Geometry check sheet. Reference: the model listing, model coordinates, mm. Give positions to 0.01 mm unless a question says otherwise; leave off trailing zeros. Write each loop counter-clockwise with the first axis right and the second up, starting at its lowest first coordinate (ties: lowest second). Pieces come first, ordered by that corner, then holes. Notation, with made-up numbers: M 41.5,36 L 54.5,36 A13 cw 54.5,54 Z; hole C 84,-3 d10. An arc over 180 degrees is marked long. One line per item, written item: value. Start each with the question number.
1. Cross-section at C-C on y = 264.5. Record the cut outline in (x, z), then the cut area to 3 significant figures.
2. Gauge pin test, flat ends, axial feed: pin 1 (10 mm diameter, centred on x = 123, z = -49.5, fed in from -Y); pin 2 (1 mm diameter, centred on x = -115, z = -49, fed in from +Y); pin 3 (3 mm diameter, centred on x = -211, z = 49.5, fed in from +Y). Record the tip position at first contact, or that the pin passes through.
3. Cross-section at A-A on z = -48.5. Record the cut outline in (x, y), then the cut area to 3 significant figures.
4. Cross-section at D-D on z = 40. Record the cut outline in (x, y), then the cut area to 3 significant figures.
5. Cross-section at B-B on x = 142. Record the cut outline in (y, z), then the cut area to 3 significant figures.
6. Scan lines: line 1 (Y direction, x = 126.5, z = 22); line 2 (Y direction, x = -320, z = -19). Record each from-to range of solid material in increasing order.
Autodesk Inventor part; units mm, degrees
ref_plane "YZ Plane" through (0, 0, 0) normal (1, 0, 0) x (0, 1, 0)
ref_plane "XZ Plane" through (0, 0, 0) normal (0, 1, 0) x (-1, 0, 0)
ref_plane "XY Plane" through (0, 0, 0) normal (0, 0, 1) x (1, 0, 0)
sketch "Sketch1" plane through (0, 0, 0) normal (0, 1, 0) x (-1, 0, 0)
  line L0 (431.8, -82.55) -> (-431.8, -82.55)
  line L1 (-431.8, -82.55) -> (-431.8, 82.55)
  line L2 (-431.8, 82.55) -> (431.8, 82.55)
  line L3 (431.8, 82.55) -> (431.8, -82.55)
  line L4 (431.8, -82.55) -> (-431.8, 82.55) construction
  line L5 (-431.8, -82.55) -> (431.8, 82.55) construction
  point P0 (0, 0)
  dimension "d0" = 863.6
  dimension "d1" = 165.1
extrude "Extrusion1" add sketch "Sketch1" along normal blind 304.8
sketch "Sketch2" plane through (431.8, 0, 82.55) normal (1, 0, 0) x (0, 0, -1)
  line L0 (0, 304.8) -> (165.1, 304.8)
  line L1 (165.1, 0) -> (165.1, 304.8)
  line L2 (12.7, 304.8) -> (165.1, 254)
  line L3 (165.1, 254) -> (165.1, 304.8)
  line L4 (165.1, 304.8) -> (12.7, 304.8)
  point P0 (82.55, 0)
  dimension "d4" = 12.7
  dimension "d5" = 50.8
extrude "Extrusion2" cut sketch "Sketch2" against normal through all
sketch "Sketch3" plane through (-431.8, 0, 82.55) normal (0, 0, 1) x (1, 0, 0)
  line L0 (0, 304.8) -> (863.6, 304.8)
  line L1 (863.6, 0) -> (863.6, 304.8)
  line L2 (431.8, 304.8) -> (431.8, 0) construction
  line L3 (863.6, 0) -> (0, 0) construction
  line L4 (711.2, 304.8) -> (863.6, 254)
  line L5 (152.4, 304.8) -> (0, 254)
  line L6 (0, 0) -> (0, 304.8)
  line L7 (0, 254) -> (0, 304.8)
  line L8 (0, 304.8) -> (152.4, 304.8)
  dimension "d8" = 152.4
  dimension "d9" = 50.8
extrude "Extrusion3" cut sketch "Sketch3" against normal through all contours L0 L1 L4
extrude "Extrusion4" cut sketch "Sketch3" against normal through all contours L0 L5 L6
properties part number "Straight_cap_7" material "Limestone"
Report:
1. outline: M -400.3,-51.05 L 400.3,-51.05 L 400.3,82.55 L -400.3,82.55 Z
1. area: 107,000 mm^2
2. pin 1: stops at y = 0
2. pin 2: stops at y = 265.35
2. pin 3: stops at y = 298.52
3. outline: M -431.8,0 L 431.8,0 L 431.8,254 L 397.75,265.35 L -397.75,265.35 L -431.8,254 Z
3. area: 229,000 mm^2
4. outline: M -431.8,0 L 431.8,0 L 431.8,254 L 309.25,294.85 L -309.25,294.85 L -431.8,254 Z
4. area: 250,000 mm^2
5. outline: M 0,-82.55 L 254,-82.55 L 304.8,69.85 L 304.8,82.55 L 0,82.55 Z
5. area: 46,500 mm^2
6. line 1: y = 0 to 288.85
6. line 2: y = 0 to 275.18
